Input: part model. Units: mm. Frame: model coordinates. Coordinates: 2 decimals unless noted, no trailing zeros. Loops run counter-clockwise (first coordinate to the right, second up) from the corner with the lowest first, then second, coordinate; pieces in that order, holes last. Notation, with made-up numbers: (-34, 7) - (0, 7) arc R24 ccw to (0, 39) - close; hole circle Ø9 at (79, 3). An arc over 180 degrees is marked (long way). Use one line per item in the form item = value.
from build123d import *

# Parameters (mm, degrees)
EXTRUDE_1_DEPTH          = 2.15
CUT_EXTRUDE_1_DEPTH      = 3
CUT_EXTRUDE_1_DEPTH_BACK = 0.8
SKETCH_3_R               = 1.5


with BuildPart() as part:
    # 草图1 → 凸台-拉伸1 (new body)
    with BuildSketch(Plane(origin=(0, 0, 0), x_dir=(1, 0, 0), z_dir=(0, 1, 0))):
        Polygon((3.175426481, 0), (1.58771324, 2.75), (-1.58771324, 2.75), (-3.175426481, 0), (-1.58771324, -2.75), (1.58771324, -2.75), align=None)
    extrude(amount=EXTRUDE_1_DEPTH)

    # 草图3 → 切除-拉伸1 (cut, two sides: drawn at the far end of the back side and taken through both)
    with BuildSketch(Plane(origin=(0, 0, 0), x_dir=(1, 0, 0), z_dir=(0, 1, 0)).offset(-CUT_EXTRUDE_1_DEPTH_BACK)):
        with Locations(Location((0, 0, 0), (0, 0, 270))):
            Circle(SKETCH_3_R)
    extrude(amount=CUT_EXTRUDE_1_DEPTH + CUT_EXTRUDE_1_DEPTH_BACK, mode=Mode.SUBTRACT)


solid = part.part
Q1. Cut plane B-B, the plane y = 0.75. Return loops of the section in (x, z).
Check values:
outline = (-3.18, 0) - (-1.59, -2.75) - (1.59, -2.75) - (3.18, 0) - (1.59, 2.75) - (-1.59, 2.75) - close; hole circle Ø3 at (0, 0)
Q2. Cut plane D-D, the plane x = 3. Return loops of the section in (y, z).
Check values:
outline = (0, -0.3) - (2.15, -0.3) - (2.15, 0.3) - (0, 0.3) - close
Q3. Ray query, line 1 along Z through (x, y) = (0, 0.85); line 2 along X through (y, z) = (0.3, 1.25); line 3 along Z through (x, y) = (-1.25, 1.4). Return the intervals inside material, ascending. Write a range as [from, to].
Check values:
line_1 = [-2.75, -1.5], [1.5, 2.75]
line_2 = [-2.45, -0.83], [0.83, 2.45]
line_3 = [-2.75, -0.83], [0.83, 2.75]
Q4. Cut plane C-C, the plane z = 1.1. Return loops of the section in (x, y).
Check values:
outline = (-2.54, 0) - (-1.02, 0) - (-1.02, 2.15) - (-2.54, 2.15) - close; (1.02, 0) - (2.54, 0) - (2.54, 2.15) - (1.02, 2.15) - close
Q5. Cut plane A-A, the plane x = 0. Return loops of the section in (y, z).
Check values:
outline = (0, -2.75) - (2.15, -2.75) - (2.15, -1.5) - (0, -1.5) - close; (0, 1.5) - (2.15, 1.5) - (2.15, 2.75) - (0, 2.75) - close
Q6. Pull-direction query (Z, two-part tool) for faces 1 (the flat face through (0, 1, -2.75)), 2 (the flat face through (2.37, 1.06, 1.394)), 3 (the cylindrical face through (0.45, 1.06, 1.43)); classes: pulls with the +Z half, pulls with the -Z half, needs draft (parallel to the pull), parting line crosses it, or undercut.
Check values:
face_1 = pulls with the -Z half
face_2 = pulls with the +Z half
face_3 = undercut
